Autodesk Inventor part; units mm, degrees
ref_plane "YZ Plane" through (0, 0, 0) normal (1, 0, 0) x (0, 1, 0)
ref_plane "XZ Plane" through (0, 0, 0) normal (0, 1, 0) x (-1, 0, 0)
ref_plane "XY Plane" through (0, 0, 0) normal (0, 0, 1) x (1, 0, 0)
sketch "Sketch1" plane through (0, 0, 0) normal (0, 1, 0) x (-1, 0, 0)
  line L0 (0, 0) -> (40, 0)
  line L1 (40, 0) -> (40, -46)
  line L2 (40, -46) -> (0, -46)
  line L3 (0, -46) -> (0, 0)
  line L4 (40, 0) -> (0, 0)
  line L5 (0, 0) -> (0, -5)
  line L6 (0, -5) -> (40, -5)
  line L7 (40, -5) -> (40, 0)
  line L8 (40, -46) -> (0, -46)
  line L9 (0, -46) -> (0, -41)
  line L10 (0, -41) -> (40, -41)
  line L11 (40, -41) -> (40, -46)
  point P0 (40, -5)
  dimension "d1" = 40
  dimension "d2" = 46
  dimension "d3" = 5
  dimension "d4" = 5
extrude "Extrusion1" add sketch "Sketch1" along normal blind 5 contours L6 L1 L10 L3
extrude "Extrusion2" add sketch "Sketch1" along normal blind 60 contours L0 L1 L6 L3 | L10 L1 L2 L3
fillet "Fillet1" radius 20 4 edges at (-40, 60, -43.5) (0, 60, -43.5) (0, 60, -2.5) (-40, 60, -2.5)
sketch "Sketch2" plane through (0, 0, -46) normal (0, 0, -1) x (-1, 0, 0)
  arc A0 (40, 40) -> (0, 40) centre (20, 40) ccw
  line L0 (0, 0) -> (0, 40)
  line L1 (0, 0) -> (40, 0)
  line L2 (40, 0) -> (40, 40)
  circle A1 centre (20, 40) radius 2.75
  point P0 (0, 0)
  dimension "d10" = 5.5
extrude "Extrusion3" cut sketch "Sketch2" against normal blind 600 contours A1
properties part number "Apoio_Fixo_3DPrint"
Build history of the part. All positions in model axes, mm. A direction names the side the tool comes from. Round coordinates to 2 decimals unless told otherwise and drop trailing zeros. Order: outer loops, then holes, each group sorted by start corner. A loop starts at its lowest first (then second) coordinate and runs counter-clockwise, first axis right, second up. Notation, with made-up numbers: M -23,-27 L 25,-27 A29 cw 25,-7 Z; hole C 8,-8.5 d7. An arc over 180 degrees is marked long. Use CSV: the item, a comma, the result in double quotes. Start each with the question number.
(1) Cut at D-D on y = 38.5. List the corners of the cut face in (x, z), then the cut area to 3 significant figures.
(2) Mould opens along Z. For faces 3 (the face through (-20, 30, -46)), 4 (the face through (-19.642, 42.727, -2.535)), 5 (the face through (-20, 32, -41)) say: +Z half, -Z half, draft (parallel to the pull), parting line (faces both ways), or undercut.
(3) Tool access for faces 1 (the face through (-20, 5, -23)), 2 (the face through (-40, 4, -21)): list every direction of +Z, -Z, +X, -X, +Y, -Y with a clear straight run to the whole face (end or side of a thin tool).
(4) Flat gauge pins, fed straight in: P1, Ø10, axis at x = -10, z = -12, coming from the +Y side; P2, Ø3.5, axis at x = -20, y = 40, coming from the -Z side. Where does each tip first touch, or does it go through?
(5) Cut at B-B on y = 7.5. List the corners of the cut face in (x, z).
(6) Cut at C-C on x = -22. List the corners of the cut face in (y, z).
(7) Drill centre lines: probe 1 along Y at (x, z) = (-20, -45); probe 2 along Z at (x, y) = (-24, 17); probe 3 along Y at (x, z) = (-15.5, -6.5). Where is each one in solid material? Low to high.
Findings:
1,outline,"M -40,-46 L -22.3,-46 L -22.3,-41 L -40,-41 Z; M -40,-5 L -22.3,-5 L -22.3,0 L -40,0 Z; M -17.7,-46 L 0,-46 L 0,-41 L -17.7,-41 Z; M -17.7,-5 L 0,-5 L 0,0 L -17.7,0 Z"
1,area,"354 mm^2"
2,face 3,"-Z half"
2,face 4,"draft"
2,face 5,"undercut"
3,face 1,"+X, -X, +Y"
3,face 2,"+Z, -Z, -X, +Y, -Y"
4,P1,"stops at y = 5"
4,P2,"passes through"
5,outline,"M -40,-46 L 0,-46 L 0,-41 L -40,-41 Z; M -40,-5 L 0,-5 L 0,0 L -40,0 Z"
6,outline,"M 0,-46 L 38.11,-46 L 38.11,-41 L 5,-41 L 5,-5 L 38.11,-5 L 38.11,0 L 0,0 Z; M 41.89,-46 L 59.9,-46 L 59.9,-41 L 41.89,-41 Z; M 41.89,-5 L 59.9,-5 L 59.9,0 L 41.89,0 Z"
7,probe 1,"y = 0 to 37.25, 42.75 to 60"
7,probe 2,"z = -46 to -41, -5 to 0"
7,probe 3,"y = 0 to 5"
